from build123d import *

# Parameters (mm, degrees)
SKETCH1_R                = 32.5
SKETCH1_R_2              = 16
SKETCH1_R_3              = 1
BOSS_EXTRUDE1_DEPTH      = 3
SKETCH2_R                = 20.5
SKETCH2_R_2              = 17.5
BOSS_EXTRUDE2_DEPTH      = 10
M4_CLEARANCE_HOLE2_D     = 4.5
M4_CLEARANCE_HOLE2_DEPTH = 11.5
M4_CLEARANCE_HOLE2_TIP   = 1.351936393
CHAMFER1_SIZE            = 0.5


with BuildPart() as part:
    # Sketch1 → Boss-Extrude1 (new body)
    with BuildSketch(Plane(origin=(0, 0, 0), x_dir=(1, 0, 0), z_dir=(0, 1, 0))):
        with Locations(Location((0, 0, 0), (0, 0, 270))):
            Circle(SKETCH1_R)
        with Locations(Location((0, 0, 0), (0, 0, 270))):
            Circle(SKETCH1_R_2, mode=Mode.SUBTRACT)
        with Locations(Location((0, 27, 0), (0, 0, 270))):
            Circle(SKETCH1_R_3, mode=Mode.SUBTRACT)
        with Locations(Location((27, 0, 0), (0, 0, 270))):
            Circle(SKETCH1_R_3, mode=Mode.SUBTRACT)
        with Locations(Location((0, -27, 0), (0, 0, 270))):
            Circle(SKETCH1_R_3, mode=Mode.SUBTRACT)
        with Locations(Location((-27, 0, 0), (0, 0, 270))):
            Circle(SKETCH1_R_3, mode=Mode.SUBTRACT)
    extrude(amount=BOSS_EXTRUDE1_DEPTH)

    # Sketch2 → Boss-Extrude2 (add)
    with BuildSketch(Plane(origin=(0, 3, 0), x_dir=(1, 0, 0), z_dir=(0, 1, 0))):
        with Locations(Location((0, 0, 0), (0, 0, 270))):
            Circle(SKETCH2_R)
        with Locations(Location((0, 0, 0), (0, 0, 270))):
            Circle(SKETCH2_R_2, mode=Mode.SUBTRACT)
    extrude(amount=BOSS_EXTRUDE2_DEPTH)

    # M4 Clearance Hole2
    with Locations(Plane(origin=(0, 3, 0), x_dir=(1, 0, 0), z_dir=(0, 1, 0))):
        with Locations((0, 27), (27, 0), (0, -27), (-27, 0)):
            Hole(M4_CLEARANCE_HOLE2_D / 2, depth=M4_CLEARANCE_HOLE2_DEPTH)
            with Locations((0, 0, -(M4_CLEARANCE_HOLE2_DEPTH + M4_CLEARANCE_HOLE2_TIP / 2))):  # 118° drill point
                Cone(0, M4_CLEARANCE_HOLE2_D / 2, M4_CLEARANCE_HOLE2_TIP, mode=Mode.SUBTRACT)

    # Chamfer1
    chamfer1_edges = [part.edges().sort_by_distance(p)[0] for p in [
        (0, 13, -20.5),
        (0, 13, -17.5),
    ]]
    chamfer(chamfer1_edges, length=CHAMFER1_SIZE)


solid = part.part
Design review of the part built by this model. Coordinates are the model's own, in mm. A direction names the side the tool comes from. Give positions to 0.01 mm unless a question says otherwise; leave off trailing zeros. Loops run counter-clockwise (first coordinate to the right, second up) from the corner with the lowest first, then second, coordinate; pieces in that order, holes last. Notation, with made-up numbers: M 63,-31 L 74,-31 A15 ccw 74,-26 Z; hole C 31.5,78.25 d4. An arc over 180 degrees is marked long. One line per question, with ' | ' between items. Start each with the question number.
1. Add section B-B (z = -27). Write out the cut boundary in (x, y), plus the area to 3 significant figures.
2. Insertion check: P1, Ø5, axis at x = -22, z = -10.5, coming from the +Y side; P2, Ø2, axis at y = 3, z = -16, coming from the +X side. Each pin has a flat end and moves straight along its axis. Give the tip position at first contact, or say it passes through.
3. To check wall thickness, follow L1, parallel to Y at x = -24, z = 6.5; L2, parallel to X at y = 9, z = 0; L3, parallel to Z at x = 27, y = 1.25. State the ranges of each line that lie inside material, in increasing order.
4. Add section D-D (y = 10.5). Write out the cut boundary in (x, z).
5. Add section C-C (x = 26). Write out the cut boundary in (y, z), plus the area to 3 significant figures.
6. For faces 1 (the face through (-20.013, 7.684, -4.444)), 2 (the face through (0.488, 1.479, 29.196)), list the 3-axis set-ups (+Z, -Z, +X, -X, +Y, -Y) from which the entire face can be reached by the end or side of a thin tool; tool diameter is ignored.
7. Add section A-A (x = 0). Write out the cut boundary in (y, z).
8. The part is to be moulded in two halves that separate along X. For faces 3 (the face through (15, 0, 7)), 4 (the face through (9.76, 1.48, 31)), 5 (the face through (-14.2, 3, 7.7)), say which applies: released by +X, released by -X, zero draft, split by the parting line, or undercut.
Worked out:
1) outline: M -18.09,0 L -2.25,0 L -2.25,3 L -18.09,3 Z; M 2.25,0 L 18.09,0 L 18.09,3 L 2.25,3 Z | area: 95.0 mm²
2) P1: stops at y = 3 | P2: stops at x = 28.83
3) L1: y = 0 to 3 | L2: x = -20.5 to -17.5, 17.5 to 20.5 | L3: z = -18.09 to -2.25, 2.25 to 18.09
4) outline: C 0,0 d41; hole C 0,0 d35
5) outline: M 0,-19.5 L 3,-19.5 L 3,-2.02 L 0,-2.02 Z; M 0,2.02 L 3,2.02 L 3,19.5 L 0,19.5 Z | area: 105 mm²
6) face 1: +Y | face 2: +Y, -Y
7) outline: M 0,-32.5 L 3,-32.5 L 3,-29.25 L 0,-29.25 Z; M 0,-24.75 L 3,-24.75 L 3,-20.5 L 12.5,-20.5 L 13,-20 L 13,-18 L 12.5,-17.5 L 3,-17.5 L 3,-16 L 0,-16 Z; M 0,16 L 3,16 L 3,17.5 L 12.5,17.5 L 13,18 L 13,20 L 12.5,20.5 L 3,20.5 L 3,24.75 L 0,24.75 Z; M 0,29.25 L 3,29.25 L 3,32.5 L 0,32.5 Z
8) face 3: zero draft | face 4: split by the parting line | face 5: undercut
